Check sheet for the modelled part. Datum: model origin and axes. Units: mm. Round coordinates to 2 decimals unless told otherwise and drop trailing zeros. Order: outer loops, then holes, each group sorted by start corner. A loop starts at its lowest first (then second) coordinate and runs counter-clockwise, first axis right, second up.
```python
from build123d import *

# Parameters (mm, degrees)
F1_DEPTH = 26.5
F2_R     = 12
F3_R     = 3


with BuildPart() as f1:
    # F0 (on Front) → F1 (new body, symmetric)
    with BuildSketch(Plane.XZ):
        with BuildLine():
            ThreePointArc((-175, 0), (0, 37.221436), (175, 0))
            Line((175, 0), (178.255814, 7.307508))
            ThreePointArc((178.255814, 7.307508), (0, 45.221436), (-178.255814, 7.307508))
            Line((-178.255814, 7.307508), (-175, 0))
        make_face()
    extrude(amount=F1_DEPTH, both=True)

    # F2
    f2_edges = [f1.edges().sort_by_distance(p)[0] for p in [
        (-176.627907, -26.5, 3.653754),
        (176.627907, -26.5, 3.653754),
    ]]
    fillet(f2_edges, radius=F2_R)

    # F3
    f3_edges = [f1.edges().sort_by_distance(p)[0] for p in [
        (175, 6, 0),
        (171.783213, -22.985785, 1.417489),
        (0, 26.5, 37.221436),
        (0, -26.5, 37.221436),
        (-175, 6, 0),
        (-171.783212, -22.985786, 1.417489),
        (178.255814, 6, 7.307508),
        (175.03915, -22.985767, 8.72523),
        (0, 26.5, 45.221436),
        (0, -26.5, 45.221436),
        (-178.255814, 6, 7.307508),
        (-175.03915, -22.985767, 8.725229),
    ]]
    fillet(f3_edges, radius=F3_R)


solid = f1.part
```
Item 1: Go/stop test with flat-tipped pins: P1, Ø4, axis at y = 4, z = 6.5, coming from the -X side; P2, Ø3, axis at y = -5.5, z = 15, coming from the -X side; P3, Ø1.5, axis at y = 20, z = 11, coming from the -X side; P4, Ø10, axis at x = -69.5, y = -16, coming from the +Z side. Record where each tip stops, or that it passes through.
Answer:
P1: stops at x = -177.29
P2: stops at x = -163.65
P3: stops at x = -171.5
P4: stops at z = 40.45
Item 2: Sectioned sample at A-A (y = 1.5). Record the cut outline in (x, z), and give its area (3 significant figures).
Answer:
outline: (-177.03, 4.56) - (-176.22, 2.73) arc R3 ccw to (-172.27, 1.2) arc R430 cw to (172.27, 1.2) arc R3 ccw to (176.22, 2.73) - (177.03, 4.56) arc R3 ccw to (175.49, 8.53) arc R438 ccw to (-175.49, 8.53) arc R3 ccw to start
area: 2,900 mm2
Item 3: Scan lines: line 1 along Z through (x, y) = (1, -18); line 2 along Z through (x, y) = (-142, 9); line 3 along Y through (x, z) = (14.5, 42.5). Record each from-to range of solid material in increasing order.
Answer:
line 1: z = 37.22 to 45.22
line 2: z = 13.1 to 21.56
line 3: y = -26.45 to 26.45
